Solid Edge part; units mm, degrees
sketch "Sketch1" plane through (0, 0, 0) normal (0, 0, 1) x (1, 0, 0)
  line L0 (-59.75, -14) -> (59.75, -14)
  line L1 (59.75, -14) -> (59.75, 14)
  line L2 (59.75, 14) -> (-59.75, 14)
  line L3 (-59.75, 14) -> (-59.75, -14)
extrude "Protrusion1" add sketch "Sketch1" against normal blind 40
sketch "Sketch2" plane through (0, -14, -20) normal (0, -1, 0) x (1, 0, 0)
  line L0 (-59.75, 20) -> (-41.25, 20)
  line L1 (-41.25, 20) -> (-41.25, 8)
  line L2 (-41.25, 8) -> (-59.75, 8)
  line L3 (-59.75, 8) -> (-59.75, 20)
extrude "ExtrudedCutout_1" cut sketch "Sketch2" against normal blind 28
sketch "Sketch3" plane through (0, -14, -20) normal (0, -1, 0) x (1, 0, 0)
  line L0 (59.75, 20) -> (41.25, 20)
  line L1 (41.25, 20) -> (41.25, 8)
  line L2 (41.25, 8) -> (59.75, 8)
  line L3 (59.75, 8) -> (59.75, 20)
extrude "ExtrudedCutout_2" cut sketch "Sketch3" against normal blind 28
sketch "Sketch4" plane through (0, -14, -20) normal (0, -1, 0) x (1, 0, 0)
  line L0 (41.25, 20) -> (35.75, 20)
  line L1 (35.75, 20) -> (41.25, 8)
  line L2 (41.25, 8) -> (41.25, 20)
extrude "ExtrudedCutout_3" cut sketch "Sketch4" against normal blind 28
sketch "Sketch5" plane through (0, -14, -20) normal (0, -1, 0) x (1, 0, 0)
  line L0 (-41.25, 20) -> (-35.75, 20)
  line L1 (-35.75, 20) -> (-41.25, 8)
  line L2 (-41.25, 8) -> (-41.25, 20)
extrude "ExtrudedCutout_4" cut sketch "Sketch5" against normal blind 28
sketch "Sketch6" plane through (59.75, 0, -26) normal (1, 0, 0) x (0, 1, 0)
  line L0 (-8.2, 26) -> (-8.2, -8)
  line L1 (-8.2, -8) -> (8.2, -8)
  line L2 (8.2, -8) -> (8.2, 26)
  line L3 (8.2, 26) -> (-8.2, 26)
extrude "ExtrudedCutout_5" cut sketch "Sketch6" against normal blind 119.5
chamfer "Chamfer_1" distance 6 angle 17 1 edges at (0, 8.2, 0) measured on face at (-38.6383, 8.2, -28.6733)
chamfer "Chamfer_2" distance 6 angle 17 1 edges at (0, -8.2, 0) measured on face at (1.195, -8.2, -5.3267)
chamfer "Chamfer_5" distance 18.5 distance2 2 1 edges at (59.75, 8.2, -23) measured on face at (-38.6383, 8.2, -29.6133)
chamfer "Chamfer_6" distance 18.5 distance2 2 1 edges at (59.75, -8.2, -23) measured on face at (-38.6383, -8.2, -10.3867)
chamfer "Chamfer_7" distance 18.5 distance2 2 1 edges at (-59.75, 8.2, -23) measured on face at (-41.9067, 8.2, -29.6133)
chamfer "Chamfer_8" distance 18.5 distance2 2 1 edges at (-59.75, 1, -34) measured on face at (-38.6383, -7.004, -34)
chamfer "Chamfer_9" distance 18.5 distance2 2 1 edges at (-59.75, -8.2, -24) measured on face at (-8.24, -8.2, -10.7)
chamfer "Chamfer_10" distance 18.5 distance2 2 1 edges at (59.75, 0, -34) measured on face at (-23.4067, -7.004, -34)
Verification items for the finished model (mm, model axes). A direction names the side the tool comes from. Coordinates: 2 decimals unless noted, no trailing zeros. Write each loop counter-clockwise with the first axis right and the second up, starting at its lowest first coordinate (ties: lowest second). Pieces come first, ordered by that corner, then holes. Notation, with made-up numbers: M 21.5,-5.75 L 47.5,-5.75 A28 cw 47.5,18.25 Z; hole C -33.75,73.5 d4. An arc over 180 degrees is marked long. One line per question, with ' | ' between items.
1) Material ranges on L1, parallel to Y at x = -11, z = -17; L2, parallel to Z at x = -23.5, y = 2.25; L3, parallel to Y at x = -44.5, z = -26, recorded low to high.
Solutions:
L1: -14 to -8.2, 8.2 to 14 | L2: -40 to -34 | L3: -14 to -8.55, 8.55 to 14
2) Access from +Z, -Z, +X, -X, +Y, -Y to the whole of each face (thin tool, end or side, straight path). Record for faces 1 (the face through (-50, -12, -12)), 2 (the face through (50, 12, -12)), 3 (the face through (0.54, 9.13, -2.96)), 4 (the face through (50.63, -9.214, -23.832)).
Solutions:
face 1: +Z, -X, +Y, -Y | face 2: +Z, +X, +Y, -Y | face 3: +Z, +X, -X | face 4: +Z, +X
3) Sectioned sample at C-C on x = -17.5. Record the cut outline in (y, z).
Solutions:
outline: M -14,-40 L 14,-40 L 14,0 L 10.03,0 L 8.2,-6 L 8.2,-34 L -8.2,-34 L -8.2,-6 L -10.03,0 L -14,0 Z
4) Sectioned sample at B-B on y = -1. Record the cut outline in (x, z), then the cut area to 3 significant figures.
Solutions:
outline: M -59.75,-40 L 59.75,-40 L 59.75,-36 L 41.25,-34 L -41.25,-34 L -59.75,-36 Z | area: 680 mm^2
5) Sectioned sample at D-D on z = -9.5. Record the cut outline in (x, y), then the cut area to 3 significant figures.
Solutions:
outline: M -40.1,-14 L 40.1,-14 L 40.1,-8.2 L -40.1,-8.2 Z; M -40.1,8.2 L 40.1,8.2 L 40.1,14 L -40.1,14 Z | area: 930 mm^2
6) Sectioned sample at A-A on z = -18. Record the cut outline in (x, y).
Solutions:
outline: M -59.75,-14 L 59.75,-14 L 59.75,-10.2 L 41.25,-8.2 L -41.25,-8.2 L -59.75,-10.2 Z; M -59.75,10.2 L -41.25,8.2 L 41.25,8.2 L 59.75,10.2 L 59.75,14 L -59.75,14 Z
7) Depth check by flat-ended pin: pin 1 Ø1.5 at (y, z) = (-10.5, -5.5) entering from +X; pin 2 Ø4.5 at (x, y) = (50, -12) entering from +Z; pin 3 Ø1 at (x, y) = (26.5, 3.5) entering from +Z. Enter the tip coordinate at first touch or a pass-through.
Solutions:
pin 1: x = 38.61 | pin 2: z = -12 | pin 3: z = -34
8) Release check for a two-part mould opening along Y. For faces 5 (the face through (1, 0, -34)), 6 (the face through (-1, -14, -20)), 7 (the face through (-38.461, -11.141, -5.916)) record: +Y half, -Y half, draft (parallel to the pull), parting line (faces both ways), or undercut.
Solutions:
face 5: undercut | face 6: -Y half | face 7: draft
